Verification items for the finished model (mm, model axes). Face numbers are marked on the shaded views. A direction names the side the tool comes from. Give positions to 0.01 mm unless a question says otherwise; leave off trailing zeros. Order: outer loops, then holes, each group sorted by start corner. A loop starts at its lowest first (then second) coordinate and runs counter-clockwise, first axis right, second up. Notation, with made-up numbers: (80, 29.25) -> (106, 29.25) arc R22 ccw to (106, 48.25) -> close; hole circle Ø10 at (-18.75, 77.5). An arc over 180 degrees is marked (long way). One line per question, with ' | ' between items. Start each with the question number.
Q1. Access from +Z, -Z, +X, -X, +Y, -Y to the whole of each face (thin tool, end or side, straight path). Record for the marked faces 1, 2 and 3.
Q2. Section check B-B on z = 12. Record the cut outline in (x, y).
Q3. Section check C-C on y = 1.75. Record the cut outline in (x, z), plus the area to 3 significant figures.
Q4. Material ranges on probe 1 along Z at (x, y) = (-2.75, -1.75); probe 2 along Y at (x, z) = (0, 19.75); probe 3 along X at (y, z) = (-1, 7.75), recorded low to high. Write a range as [from, to].
Q5. Section check A-A on x = 0. Record the cut outline in (y, z), plus the area to 3 significant figures.
Q6. Go/stop test with flat-tipped pins: pin 1 (2 mm diameter, centred on x = -1.5, z = 15.5, fed in from -Y); pin 2 (1 mm diameter, centred on y = -2, z = 19.5, fed in from -X); pin 3 (1.3 mm diameter, centred on x = -2, z = 13, fed in from +Y). Record where each tip stops, or that it passes through.
Q7. Mould release check, pull along Z, two halves, no side actions. Record for the marked faces 4, 5 and 6: released by +Z, released by -Z, zero draft, split by the parting line, or undercut.
Q8. Section check D-D on x = -2.75. Record the cut outline in (y, z), plus the area to 3 significant figures.
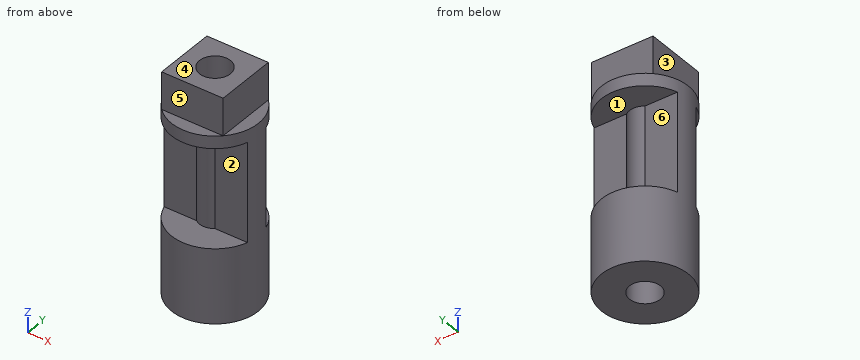
from build123d import *

# Parameters (mm, degrees)
BOSS_EXTRUDE1_START = 5
SKETCH3_R           = 3.5
SKETCH3_R_2         = 1.25
BOSS_EXTRUDE1_DEPTH = 18
SKETCH4_W           = 8
SKETCH4_H           = 2.5
CUT_EXTRUDE1_DEPTH  = 4.5
SKETCH5_OUTSIDE_W   = 13.108
SKETCH5_OUTSIDE_H   = 13.108
SKETCH5_OUTSIDE_W_2 = 4.949747468
SKETCH5_OUTSIDE_H_2 = 4.949747468
CUT_EXTRUDE2_DEPTH  = 3


with BuildPart() as part:
    # Sketch3 → Boss-Extrude1 (new body)
    with BuildSketch(Plane.XY.offset(BOSS_EXTRUDE1_START)):
        Circle(SKETCH3_R)
        Circle(SKETCH3_R_2, mode=Mode.SUBTRACT)
    extrude(amount=BOSS_EXTRUDE1_DEPTH)

    # Sketch4 → Cut-Extrude1 (cut, symmetric)
    with BuildSketch(Plane(origin=(0, 0, 0), x_dir=(0, 0, -1), z_dir=(1, 0, 0))):
        with Locations((-15, 2.25)):
            Rectangle(SKETCH4_W, SKETCH4_H)
    cut_extrude1 = extrude(amount=CUT_EXTRUDE1_DEPTH, both=True, mode=Mode.SUBTRACT)

    # Mirror1: Cut-Extrude1 across plane
    add(cut_extrude1.mirror(Plane.ZX), mode=Mode.SUBTRACT)

    # Sketch5 outside → Cut-Extrude2 (cut)
    with BuildSketch(Plane.XY.offset(23)):
        Rectangle(SKETCH5_OUTSIDE_W, SKETCH5_OUTSIDE_H)
        Rectangle(SKETCH5_OUTSIDE_W_2, SKETCH5_OUTSIDE_H_2, mode=Mode.SUBTRACT)
    extrude(amount=-CUT_EXTRUDE2_DEPTH, mode=Mode.SUBTRACT)


solid = part.part
Filled in:
1) face 1: +X, -X, +Y | face 2: +X, -X, -Y | face 3: +Z, -X, +Y, -Y
2) outline: (-3.35, -1) -> (-0.75, -1) arc R1.25 cw to (-0.75, 1) -> (-3.35, 1) arc R3.5 ccw to start; (0.75, -1) -> (3.35, -1) arc R3.5 ccw to (3.35, 1) -> (0.75, 1) arc R1.25 cw to start
3) outline: (-3.03, 5) -> (3.03, 5) -> (3.03, 11) -> (-3.03, 11) -> close; (-3.03, 19) -> (3.03, 19) -> (3.03, 20) -> (2.47, 20) -> (2.47, 23) -> (-2.47, 23) -> (-2.47, 20) -> (-3.03, 20) -> close | area: 57.3 mm²
4) probe 1: [5, 11], [19, 20] | probe 2: [-3.5, -1.25], [1.25, 3.5] | probe 3: [-3.35, -0.75], [0.75, 3.35]
5) outline: (-3.5, 5) -> (-1.25, 5) -> (-1.25, 11) -> (-3.5, 11) -> close; (-3.5, 19) -> (-1.25, 19) -> (-1.25, 23) -> (-2.47, 23) -> (-2.47, 20) -> (-3.5, 20) -> close; (1.25, 5) -> (3.5, 5) -> (3.5, 11) -> (1.25, 11) -> close; (1.25, 19) -> (3.5, 19) -> (3.5, 20) -> (2.47, 20) -> (2.47, 23) -> (1.25, 23) -> close | area: 38.8 mm²
6) pin 1: y = -1 | pin 2: x = -3.16 | pin 3: y = 1
7) face 4: released by +Z | face 5: zero draft | face 6: undercut
8) outline: (-2.17, 5) -> (2.17, 5) -> (2.17, 11) -> (1, 11) -> (1, 19) -> (2.17, 19) -> (2.17, 20) -> (-2.17, 20) -> (-2.17, 19) -> (-1, 19) -> (-1, 11) -> (-2.17, 11) -> close | area: 46.3 mm²
